Here's the drawing with two shaded views (mm, measured from the low corner). I have some questions. A direction names the side the tool comes from. Round coordinates to 2 decimals unless told otherwise and drop trailing zeros. Loops run counter-clockwise (first coordinate to the right, second up) from the corner with the lowest first, then second, coordinate; pieces in that order, holes last. Notation, with made-up numbers: M 28.25,-39 L 82.25,-39 A25 cw 82.25,-16 Z; hole C 30,22 d2. An arc over 180 degrees is marked long. One line per item, written item: value. Start each with the question number.
Q1. Imagine slicing it at D-D (z = 434). Please give me the cut outline in (x, y), then the cut area to 3 significant figures.
Q2. Imagine slicing it at B-B (z = 69). Please give me the cut outline in (x, y).
Q3. Which directions (+Z, -Z, +X, -X, +Y, -Y) give clear straight access to the entire face, cutting with the end or side of a thin tool? Please do the marked faces 1 and 2.
Q4. Imagine slicing it at C-C (y = 328). Please give me the cut outline in (x, z), then the cut area to 3 significant figures.
Q5. Imagine slicing it at A-A (x = 300). Please give me the cut outline in (y, z).
Q6. Thinking about a two-plate mould opening in Y: for the marked faces 3, 4 and 5, which applies, released by +Y, released by -Y, zero draft, split by the parting line, or undercut?
Q7. Please list where these lines run through material, in increasing order: line 1 along Y through (x, z) = (200, 58); line 2 along X through (y, z) = (125, 49); line 3 along Z through (x, y) = (300, 417).
Q8. I'm going to push flat-ended pins straight in: pin 1 Ø12 at (x, y) = (337, 153) entering from +Z; pin 2 Ø10 at (x, z) = (315, 256.5) entering from -Y. Where does each tip first touch, or does it pass through?
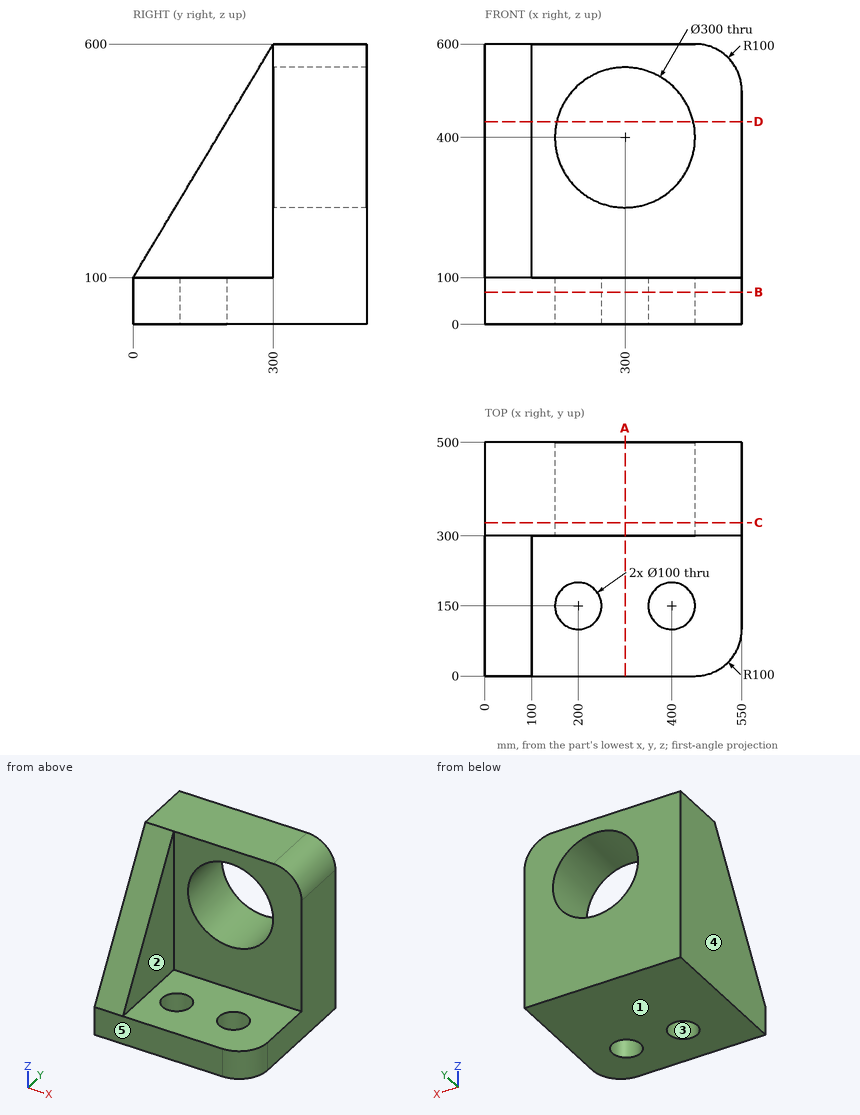
Report:
1. outline: M 0,200.4 L 100,200.4 L 100,300 L 153.9,300 L 153.9,500 L 0,500 Z; M 446.1,300 L 550,300 L 550,500 L 446.1,500 Z
1. area: 61,500 mm²
2. outline: M 0,0 L 450,0 A100 ccw 550,100 L 550,500 L 0,500 Z; hole C 200,150 d100; hole C 400,150 d100
3. face 1: -Z, +X, -X, +Y, -Y
3. face 2: +Z, +X, -Y
4. outline: M 0,0 L 550,0 L 550,500 A100 ccw 450,600 L 0,600 Z; hole C 300,400 d300
4. area: 257,000 mm²
5. outline: M 0,0 L 500,0 L 500,250 L 300,250 L 300,100 L 0,100 Z; M 300,550 L 500,550 L 500,600 L 300,600 Z
6. face 3: undercut
6. face 4: zero draft
6. face 5: released by -Y
7. line 1: y = 0 to 100, 200 to 500
7. line 2: x = 0 to 156.7, 243.3 to 356.7, 443.3 to 550
7. line 3: z = 0 to 250, 550 to 600
8. pin 1: stops at z = 100
8. pin 2: passes through
